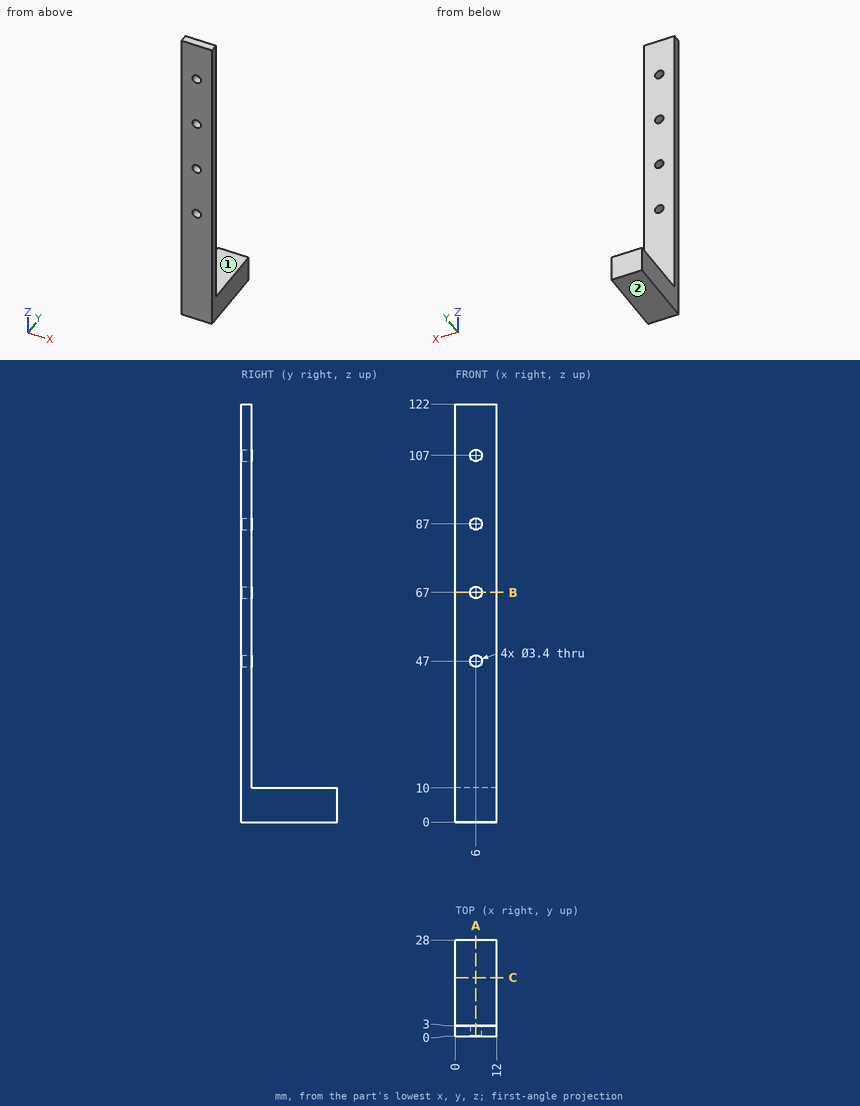
Part print with two shaded views. Sizes in mm from the minimum x, y, z corner. A direction names the side the tool comes from. Coordinates: 2 decimals unless noted, no trailing zeros. Write each loop counter-clockwise with the first axis right and the second up, starting at its lowest first coordinate (ties: lowest second). Pieces come first, ordered by that corner, then holes.
1. Drop flat-ended pins along their axis: pin 1 (3 mm diameter, centred on x = 5, y = 12, fed in from +Z); pin 2 (3.5 mm diameter, centred on x = 6.5, z = 83, fed in from +Y); pin 3 (2.5 mm diameter, centred on x = 6, z = 67, fed in from +Y). Give the stop position or say it passes through.
Answer block:
pin 1: stops at z = 10
pin 2: stops at y = 3
pin 3: passes through
2. Band-saw the part on C-C, the plane y = 17. Give the cut face in (x, z), and give its area (3 significant figures).
Answer block:
outline: (0, 0) - (12, 0) - (12, 10) - (0, 10) - close
area: 120 mm2
3. Drill centre lines: probe 1 along Z at (x, y) = (6, 1.9); probe 2 along Z at (x, y) = (8, 14.25); probe 3 along Y at (x, z) = (3.75, 70.5). Where is each one in solid material? Low to high.
Answer block:
probe 1: z = 0 to 45.3, 48.7 to 65.3, 68.7 to 85.3, 88.7 to 105.3, 108.7 to 122
probe 2: z = 0 to 10
probe 3: y = 0 to 3
4. Band-saw the part on B-B, the plane z = 67. Give the cut face in (x, y).
Answer block:
outline: (0, 0) - (4.3, 0) - (4.3, 3) - (0, 3) - close; (7.7, 0) - (12, 0) - (12, 3) - (7.7, 3) - close
5. 3-axis set-ups, long thin cutter, end or side, ignore diameter. For the marked faces 1 and 2: which of +Z, -Z, +X, -X, +Y, -Y reach the whole face in a straight line?
Answer block:
face 1: +Z, +X, -X, +Y
face 2: -Z, +X, -X, +Y, -Y
6. Band-saw the part on A-A, the plane x = 6. Give the cut face in (y, z).
Answer block:
outline: (0, 0) - (28, 0) - (28, 10) - (3, 10) - (3, 45.3) - (0, 45.3) - close; (0, 48.7) - (3, 48.7) - (3, 65.3) - (0, 65.3) - close; (0, 68.7) - (3, 68.7) - (3, 85.3) - (0, 85.3) - close; (0, 88.7) - (3, 88.7) - (3, 105.3) - (0, 105.3) - close; (0, 108.7) - (3, 108.7) - (3, 122) - (0, 122) - close
